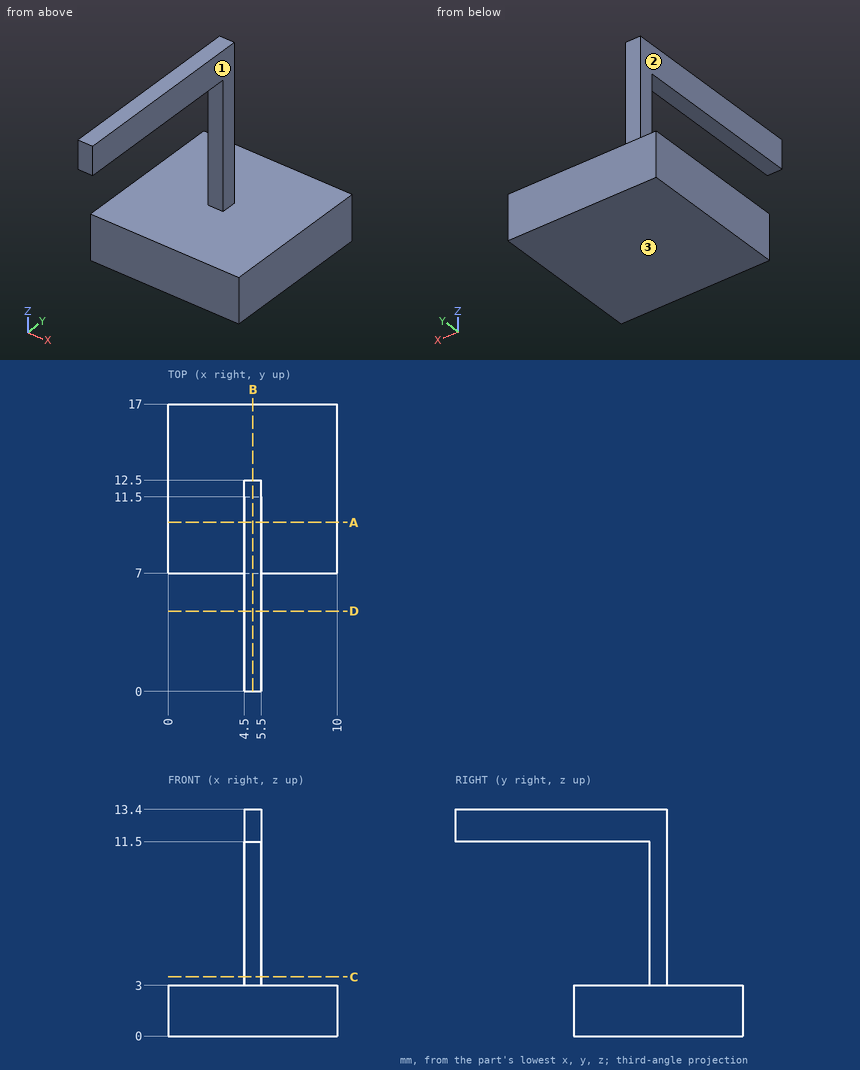
Print and shaded views of the part. All mm, measured from the part's lowest x, y and z. A direction names the side the tool comes from. Coordinates: 2 decimals unless noted, no trailing zeros. Order: outer loops, then holes, each group sorted by start corner. A loop starts at its lowest first (then second) coordinate and runs counter-clockwise, first axis right, second up. Notation, with made-up numbers: (-21, 87.25) -> (-11, 87.25) arc R24 cw to (-11, 106.25) -> close; hole circle Ø1 at (88.25, -13.5). An arc over 180 degrees is marked (long way). Answer as a JSON object with one key per item and string values. Group by question number.
1) Cut at C-C, the plane z = 3.5. Write the cut outline in (x, y).
2) Drill centre lines: L1, parallel to Y at x = 4, z = 2.25; L2, parallel to Z at x = 6.75, y = 8.5; L3, parallel to X at y = 8.5, z = 12.5. Where is each one in solid material? Low to high.
3) Which spindle directions (+Z, -Z, +X, -X, +Y, -Y) get a long thin tool onto all of the face, cutting with end or side? Do the marked faces 1, 2 and 3. Say none if no direction does.
4) Flat gauge pins, fed straight in: pin 1 (2 mm diameter, centred on x = 2, z = 6.5, fed in from -Y); pin 2 (1.5 mm diameter, centred on x = 1, y = 11.5, fed in from +Z); pin 3 (2.5 mm diameter, centred on x = 5, z = 1.5, fed in from -Y); pin 4 (0.5 mm diameter, centred on x = 5, z = 7.5, fed in from -Y). Where does each tip first touch, or does it go through?
5) Cut at D-D, the plane y = 4.75. Write the cut outline in (x, z), then the cut area to 3 significant figures.
6) Cut at A-A, the plane y = 10. Write the cut outline in (x, z).
7) Cut at B-B, the plane x = 5. Write the cut outline in (y, z).
Check values:
{
 "1": {"outline": "(4.5, 11.5) -> (5.5, 11.5) -> (5.5, 12.5) -> (4.5, 12.5) -> close"},
 "2": {"L1": "y = 7 to 17", "L2": "z = 0 to 3", "L3": "x = 4.5 to 5.5"},
 "3": {"face 1": "+Z, +X, +Y, -Y", "face 2": "+Z, -X, +Y, -Y", "face 3": "-Z, +X, -X, +Y, -Y"},
 "4": {"pin 1": "passes through", "pin 2": "stops at z = 3", "pin 3": "stops at y = 7", "pin 4": "stops at y = 11.5"},
 "5": {"outline": "(4.5, 11.5) -> (5.5, 11.5) -> (5.5, 13.4) -> (4.5, 13.4) -> close", "area": "1.90 mm²"},
 "6": {"outline": "(0, 0) -> (10, 0) -> (10, 3) -> (0, 3) -> close; (4.5, 11.5) -> (5.5, 11.5) -> (5.5, 13.4) -> (4.5, 13.4) -> close"},
 "7": {"outline": "(0, 11.5) -> (11.5, 11.5) -> (11.5, 3) -> (7, 3) -> (7, 0) -> (17, 0) -> (17, 3) -> (12.5, 3) -> (12.5, 13.4) -> (0, 13.4) -> close"}
}
